Autodesk Inventor part; units mm, degrees
ref_plane "YZ Plane" through (0, 0, 0) normal (1, 0, 0) x (0, 1, 0)
ref_plane "XZ Plane" through (0, 0, 0) normal (0, 1, 0) x (-1, 0, 0)
ref_plane "XY Plane" through (0, 0, 0) normal (0, 0, 1) x (1, 0, 0)
sketch "Sketch1" plane through (0, 0, 0) normal (0, 0, 1) x (1, 0, 0)
  line L0 (0, 0) -> (100, 0)
  line L1 (100, 0) -> (100, 59)
  line L2 (100, 59) -> (0, 59)
  line L3 (0, 59) -> (0, 0)
  dimension "d0" = 100
  dimension "d1" = 59
extrude "Extrusion1" add sketch "Sketch1" along normal blind 5
sketch "Sketch2" plane through (0, 0, 5) normal (0, 0, 1) x (1, 0, 0)
  line L0 (0, 0) -> (100, 0)
  line L1 (100, 59) -> (0, 59)
  line L2 (79.5, 0) -> (20.5, 0)
  line L3 (20.5, 0) -> (20.5, 59)
  line L4 (20.5, 59) -> (79.5, 59)
  line L5 (79.5, 59) -> (79.5, 0)
  line L6 (76.5, 3) -> (23.5, 3)
  line L7 (23.5, 3) -> (23.5, 56)
  line L8 (23.5, 56) -> (76.5, 56)
  line L9 (76.5, 56) -> (76.5, 3)
  line L10 (100, 0) -> (100, 59)
  point P0 (79.5, 59)
  point P1 (20.5, 0)
  dimension "d4" = 59
  dimension "d5" = 53
  dimension "d6" = 3
  dimension "d7" = 3
  dimension "d8" = 3
  dimension "d9" = 20.5
extrude "Extrusion2" add sketch "Sketch2" along normal blind 25 contours L3 L1 L5 L0
chamfer "Chamfer1" distance 2 angle 45 1 edges at (50, 3, 30)
chamfer "Chamfer2" distance 2 angle 45 1 edges at (76.5, 29.5, 30)
chamfer "Chamfer3" distance 2 angle 45 2 edges at (50, 56, 30) (23.5, 29.5, 30)
sketch "Sketch3" plane through (0, 0, 5) normal (0, 0, 1) x (1, 0, 0)
  circle A0 centre (87.5, 17) radius 3.25
  circle A1 centre (87.5, 42) radius 3.25
  line L0 (100, 0) -> (100, 59)
  line L1 (0, 0) -> (100, 0)
  line L2 (50, -16.6248) -> (50, 70.7208)
  line L3 (0, 59) -> (0, 0)
  circle A2 centre (12.5, 17) radius 3.25
  circle A3 centre (12.5, 42) radius 3.25
  point P0 (79.5, 0)
  dimension "d21" = 6.5
  dimension "d22" = 6.5
  dimension "d23" = 12.5
  dimension "d24" = 12.5
  dimension "d25" = 25
  dimension "d26" = 17
  dimension "d27" = 50
extrude "Extrusion3" cut sketch "Sketch3" against normal blind 60
fillet "Fillet1" radius 2 2 edges at (20.5, 29.5, 5) (79.5, 29.5, 5)
fillet "Fillet2" radius 2 2 edges at (0, 29.5, 5) (100, 29.5, 5)
fillet "Fillet3" radius 2 20 edges at (20.5, 0, 18.5) (19.9142, 0, 5.5858) (10.25, 0, 5) (0.5858, 0, 4.4142) (0, 0, 1.5) (79.5, 0, 18.5) (80.0858, 0, 5.5858) (89.75, 0, 5) (99.4142, 0, 4.4142) (100, 0, 1.5) (79.5, 59, 18.5) (80.0858, 59, 5.5858) (89.75, 59, 5) (99.4142, 59, 4.4142) (100, 59, 1.5) (20.5, 59, 18.5) (19.9142, 59, 5.5858) (10.25, 59, 5) (0.5858, 59, 4.4142) (0, 59, 1.5)
properties part number "trypsinHolder"
Model file for the job. Use its own axes, mm. A direction names the side the tool comes from. Give positions to 0.01 mm unless a question says otherwise; leave off trailing zeros. Write each loop counter-clockwise with the first axis right and the second up, starting at its lowest first coordinate (ties: lowest second). Pieces come first, ordered by that corner, then holes. Notation, with made-up numbers: (14, 75) - (48, 75) arc R32 cw to (48, 111) - close; hole circle Ø4 at (37.5, 17.5). An arc over 180 degrees is marked (long way). Answer as CSV lines item,"result".
1. Pin check, flat tips, straight feed: pin 1 (5 mm diameter, centred on x = 12.5, y = 42, fed in from -Z); pin 2 (7 mm diameter, centred on y = 35.5, z = 13, fed in from -X); pin 3 (1.5 mm diameter, centred on x = 30.5, y = 25.5, fed in from +Z); pin 4 (7 mm diameter, centred on y = 16.5, z = 19.5, fed in from +X). Stop position of each tip, or through.
Responses:
pin 1,"passes through"
pin 2,"stops at x = 20.5"
pin 3,"stops at z = 5"
pin 4,"stops at x = 79.5"
2. Band-saw the part on C-C (z = 21.5). Write the cut outline in (x, y).
Responses:
outline,"(20.5, 2) arc R2 ccw to (22.5, 0) - (77.5, 0) arc R2 ccw to (79.5, 2) - (79.5, 57) arc R2 ccw to (77.5, 59) - (22.5, 59) arc R2 ccw to (20.5, 57) - close; hole (23.5, 3) - (76.5, 3) - (76.5, 56) - (23.5, 56) - close"
3. 3-axis set-ups, long thin cutter, end or side, ignore diameter. For faces 4 (the face through (20.5, 29, 18)), 5 (the face through (76.5, 30, 16)), 6 (the face through (79.5, 30, 18)), 7 (the face through (78.93, 58.4, 18.66)), 8 (the face through (21.07, 0.6, 18.66)): which of +Z, -Z, +X, -X, +Y, -Y reach the whole face in a straight line?
Responses:
face 4,"+Z, -X, +Y, -Y"
face 5,"+Z"
face 6,"+Z, +X, +Y, -Y"
face 7,"+Z, +X, +Y"
face 8,"+Z, -X, -Y"
4. Band-saw the part on D-D (y = 31). Write the cut outline in (x, z).
Responses:
outline,"(0, 0) - (100, 0) - (100, 3) arc R2 ccw to (98, 5) - (81.5, 5) arc R2 cw to (79.5, 7) - (79.5, 30) - (78.5, 30) - (76.5, 28) - (76.5, 5) - (23.5, 5) - (23.5, 28) - (21.5, 30) - (20.5, 30) - (20.5, 7) arc R2 cw to (18.5, 5) - (2, 5) arc R2 ccw to (0, 3) - close"
5. Band-saw the part on A-A (x = 12.5). Write the cut outline in (y, z), and give its area (3 significant figures).
Responses:
outline,"(0, 0) - (13.75, 0) - (13.75, 5) - (2, 5) arc R2 ccw to (0, 3) - close; (20.25, 0) - (38.75, 0) - (38.75, 5) - (20.25, 5) - close; (45.25, 0) - (59, 0) - (59, 3) arc R2 ccw to (57, 5) - (45.25, 5) - close"
area,"228 mm2"
6. Drill centre lines: L1, parallel to Y at x = 12.5, z = 2.3; L2, parallel to X at y = 48.5, z = 16.5; L3, parallel to Y at x = 74.5, z = 16. Where is each one in solid material? Low to high. Write a range as [from, to].
Responses:
L1,"y = [0, 13.75], [20.25, 38.75], [45.25, 59]"
L2,"x = [20.5, 23.5], [76.5, 79.5]"
L3,"y = [0, 3], [56, 59]"
7. Band-saw the part on B-B (y = 17). Write the cut outline in (x, z).
Responses:
outline,"(0, 0) - (9.25, 0) - (9.25, 5) - (2, 5) arc R2 ccw to (0, 3) - close; (15.75, 0) - (84.25, 0) - (84.25, 5) - (81.5, 5) arc R2 cw to (79.5, 7) - (79.5, 30) - (78.5, 30) - (76.5, 28) - (76.5, 5) - (23.5, 5) - (23.5, 28) - (21.5, 30) - (20.5, 30) - (20.5, 7) arc R2 cw to (18.5, 5) - (15.75, 5) - close; (90.75, 0) - (100, 0) - (100, 3) arc R2 ccw to (98, 5) - (90.75, 5) - close"
8. Two-plate mould, pull along X, no slides. Class faces 1 (the face through (50, 56, 16)), 2 (the face through (49, 30, 0)), 3 (the face through (78.9, 0.57, 18.66)): +X half, -X half, draft (parallel to the pull), parting line (faces both ways), or undercut.
Responses:
face 1,"undercut"
face 2,"draft"
face 3,"+X half"
